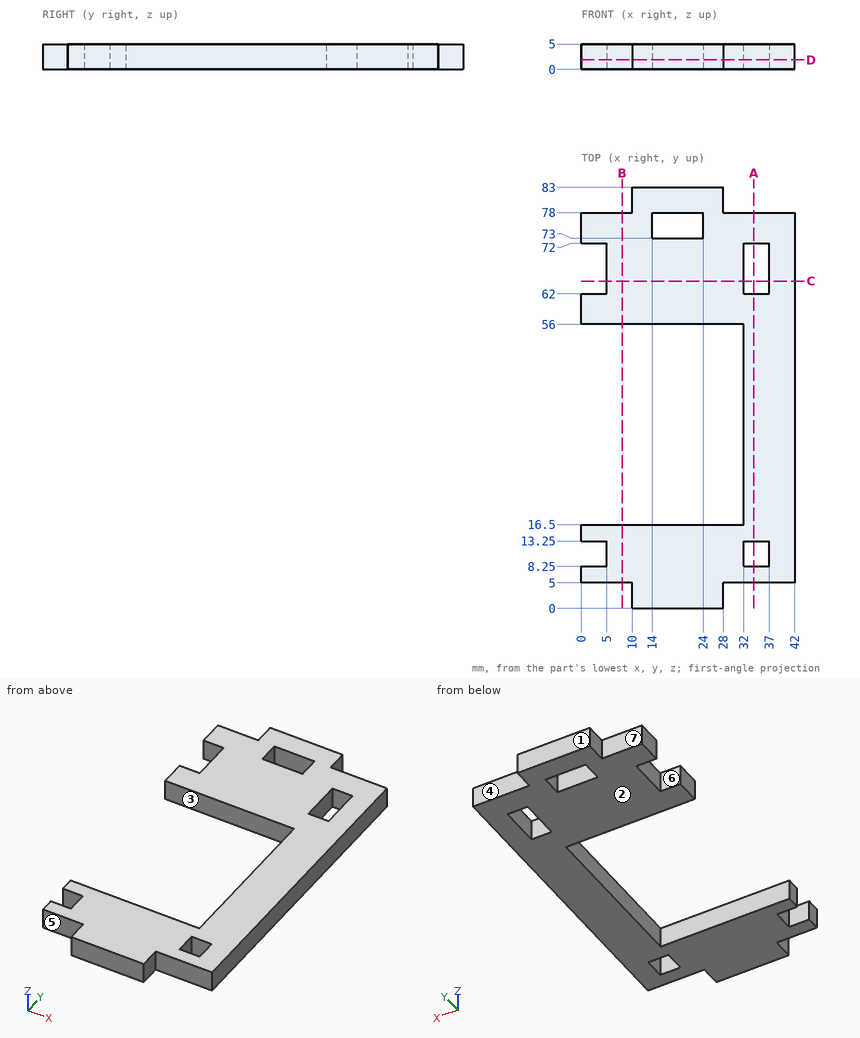
Geometry check sheet. Reference: drawing and pictorial views, mm from the part's lowest x, y, z. A direction names the side the tool comes from. Give positions to 0.01 mm unless a question says otherwise; leave off trailing zeros. Order: outer loops, then holes, each group sorted by start corner. A loop starts at its lowest first (then second) coordinate and runs counter-clockwise, first axis right, second up.
1. Thickness scan on L1, parallel to Y at x = 14.5, z = 0.75; L2, parallel to Y at x = 8, z = 2.2; L3, parallel to Y at x = 34.5, z = 3.75. Record the ranges inside material, lowest first.
2. Section check D-D, the plane z = 1.85. Give the number of separate pieces and of enclosed holes in the cut face, and give its area (3 significant figures).
3. Section check B-B, the plane x = 8. Enter the section's corners in (y, z).
4. Section check C-C, the plane y = 64.5. Enter the section's corners in (x, z), and give its area (3 significant figures).
5. Access from +Z, -Z, +X, -X, +Y, -Y to the whole of each face (thin tool, end or side, straight path). Record for the marked faces 4, 5, 6 and 7.
6. Release check for a two-part mould opening along Y. For the marked faces 1, 2 and 3 record: pulls with the +Y half, pulls with the -Y half, needs draft (parallel to the pull), parting line crosses it, or undercut.
7. Gauge pin test, flat ends, axial feed: pin 1 Ø2.5 at (x, z) = (3.5, 1.5) entering from +Y; pin 2 Ø2.5 at (y, z) = (3.5, 1.5) entering from -X; pin 3 Ø2 at (y, z) = (29, 3.5) entering from -X. Record the tip position at first contact, or that the pin passes through.
8. Section check A-A, the plane x = 34. Enter the section's corners in (y, z).
Values follow:
1. L1: y = 0 to 16.5, 56 to 73, 78 to 83
1. L2: y = 5 to 16.5, 56 to 78
1. L3: y = 5 to 8.25, 13.25 to 62, 72 to 78
2. separate pieces: 1
2. enclosed holes: 3
2. area: 1,780 mm2
3. outline: (5, 0) - (16.5, 0) - (16.5, 5) - (5, 5) - close; (56, 0) - (78, 0) - (78, 5) - (56, 5) - close
4. outline: (5, 0) - (32, 0) - (32, 5) - (5, 5) - close; (37, 0) - (42, 0) - (42, 5) - (37, 5) - close
4. area: 160 mm2
5. face 4: +Z, -Z, +X, +Y
5. face 5: +Z, -Z, -X, -Y
5. face 6: +Z, -Z, -X
5. face 7: +Z, -Z, -X, +Y
6. face 1: pulls with the +Y half
6. face 2: needs draft
6. face 3: undercut
7. pin 1: stops at y = 78
7. pin 2: stops at x = 10
7. pin 3: stops at x = 32
8. outline: (5, 0) - (8.25, 0) - (8.25, 5) - (5, 5) - close; (13.25, 0) - (62, 0) - (62, 5) - (13.25, 5) - close; (72, 0) - (78, 0) - (78, 5) - (72, 5) - close
